from build123d import *

# Parameters (mm, degrees)
CROQUIS1_W                  = 11
CROQUIS1_H                  = 10
SALIENTE_EXTRUIR1_DEPTH     = 4
CROQUIS2_R                  = 0.5
CORTAR_EXTRUIR1_DEPTH       = 12
CROQUIS3_W                  = 8
CROQUIS3_H                  = 1.977477592
CORTAR_EXTRUIR2_DEPTH       = 2
REDONDEO6_R                 = 0.5
REDONDEO8_R                 = 0.5
CORTAR_EXTRUIR3_DEPTH       = 20
CROQUIS5_W                  = 0.5
CROQUIS5_H                  = 1.744690478
CORTAR_EXTRUIR4_DEPTH       = 1
CORTAR_EXTRUIR6_DEPTH       = 12
CORTAR_EXTRUIR6_DEPTH_BACK  = 5
CROQUIS7_W                  = 1
CROQUIS7_H                  = 0.747728434
CROQUIS7_H_2                = 0.24923361
CROQUIS9_W                  = 2
CROQUIS9_H                  = 2
CORTAR_EXTRUIR7_DEPTH       = 1
REDONDEO10_R                = 0.25
CROQUIS11_W                 = 1.5
CROQUIS11_H                 = 1
CROQUIS11_W_2               = 0.5
CROQUIS11_W_3               = 1
REVOLUCI_N5_ANGLE           = 32.23
REVOLUCI_N5_OTHER_WAY_ANGLE = 0.01
CORTAR_EXTRUIR13_DEPTH      = 7
CORTAR_EXTRUIR13_DEPTH_BACK = 10
CROQUIS13_W                 = 2
CROQUIS13_H                 = 2
CORTAR_REVOLUCI_N1_ANGLE    = 5.013380707
CROQUIS15_W                 = 1
CROQUIS15_H                 = 2
REVOLUCI_N6_ANGLE           = 0.716197243
REDONDEO11_R                = 0.5
CROQUIS16_W                 = 2.973519437
CROQUIS16_H                 = 1
CROQUIS16_W_2               = 3
REVOLUCI_N7_ANGLE           = 1.432394488


with BuildPart() as part:
    # Croquis1 → Saliente-Extruir1 (new body)
    with BuildSketch(Plane(origin=(0, 0, 0), x_dir=(1, 0, 0), z_dir=(0, 1, 0))):
        with Locations((44.686928434, -17.152823879)):
            Rectangle(CROQUIS1_W, CROQUIS1_H)
    extrude(amount=SALIENTE_EXTRUIR1_DEPTH)

    # Croquis2 → Cortar-Extruir1 (cut)
    with BuildSketch(Plane.ZY.offset(-39.186928434)):
        with Locations((15.152823879, 2)):
            Circle(CROQUIS2_R)
    extrude(amount=-CORTAR_EXTRUIR1_DEPTH, mode=Mode.SUBTRACT)

    # Croquis3 → Cortar-Extruir2 (cut)
    with BuildSketch(Plane(origin=(0, 4, 0), x_dir=(1, 0, 0), z_dir=(0, 1, 0))):
        with Locations((44.686928434, -20.164085083)):
            Rectangle(CROQUIS3_W, CROQUIS3_H)
    extrude(amount=-CORTAR_EXTRUIR2_DEPTH, mode=Mode.SUBTRACT)

    # Redondeo6
    redondeo6_edges = [part.edges().sort_by_distance(p)[0] for p in [
        (48.686928434, 3, 19.175346287),
        (48.686928434, 3, 21.152823879),
        (40.686928434, 3, 21.152823879),
        (40.686928434, 3, 19.175346287),
    ]]
    fillet(redondeo6_edges, radius=REDONDEO6_R)

    # Redondeo8
    redondeo8_edges = [part.edges().sort_by_distance(p)[0] for p in [
        (44.686928434, 2, 19.175346287),
        (48.686928434, 2, 20.164085083),
        (40.686928434, 2, 20.164085083),
        (44.686928434, 2, 21.152823879),
        (40.833375043, 2, 19.321792897),
        (40.833375043, 2, 21.00637727),
        (48.540481825, 2, 21.00637727),
        (48.540481825, 2, 19.321792897),
    ]]
    fillet(redondeo8_edges, radius=REDONDEO8_R)

    # Croquis4 → Cortar-Extruir3 (cut)
    with BuildSketch(Plane(origin=(50.186928434, 0, 0), x_dir=(0, 0, -1), z_dir=(1, 0, 0))):
        with BuildLine():
            Line((-12.152823879, 4), (-13.897514357, 4))
            ThreePointArc((-13.897514357, 4), (-12.727134054, 3.425689825), (-12.152823879, 2.255309522))
            Line((-12.152823879, 2.255309522), (-12.152823879, 4))
        make_face()
        with BuildLine():
            ThreePointArc((-12.152823879, 1.744690478), (-12.727134054, 0.574310175), (-13.897514357, 0))
            Line((-13.897514357, 0), (-12.152823879, 0))
            Line((-12.152823879, 0), (-12.152823879, 1.744690478))
        make_face()
    extrude(amount=-CORTAR_EXTRUIR3_DEPTH, mode=Mode.SUBTRACT)

    # Croquis5 → Cortar-Extruir4 (cut)
    with BuildSketch(Plane.XZ):
        Polygon((44.686928434, 13.897514357), (44.686928434, 17.970046761), (44.686928434, 20.152823879), (44.186928434, 20.152823879), (44.186928434, 13.897514357), align=None)
        Polygon((44.686928434, 20.152823879), (44.686928434, 17.970046761), (44.686928434, 13.897514357), (45.186928434, 13.897514357), (45.186928434, 20.152823879), align=None)
        with Locations((44.436928434, 13.025169118)):
            Rectangle(CROQUIS5_W, CROQUIS5_H)
        with Locations((44.936928434, 13.025169118)):
            Rectangle(CROQUIS5_W, CROQUIS5_H)
    extrude(amount=-CORTAR_EXTRUIR4_DEPTH, mode=Mode.SUBTRACT)

    # Croquis7 → Cortar-Extruir6 (cut, two sides: drawn at the far end of the back side and taken through both)
    with BuildSketch(Plane.XZ.offset(-1).offset(-CORTAR_EXTRUIR6_DEPTH_BACK)):
        with Locations((44.686928434, 12.775921706)):
            Rectangle(CROQUIS7_W, CROQUIS7_H)
        with Locations((44.686928434, 12.277440684)):
            Rectangle(CROQUIS7_W, CROQUIS7_H_2)
    extrude(amount=CORTAR_EXTRUIR6_DEPTH + CORTAR_EXTRUIR6_DEPTH_BACK, mode=Mode.SUBTRACT)

    # Croquis9 → Cortar-Extruir7 (cut)
    with BuildSketch(Plane.XZ):
        with Locations((44.686928434, 21.152823879)):
            Rectangle(CROQUIS9_W, CROQUIS9_H)
    extrude(amount=-CORTAR_EXTRUIR7_DEPTH, mode=Mode.SUBTRACT)

    # Redondeo10
    redondeo10_edges = [part.edges().sort_by_distance(p)[0] for p in [
        (45.686928434, 0.5, 20.152823879),
        (43.686928434, 0.5, 20.152823879),
    ]]
    fillet(redondeo10_edges, radius=REDONDEO10_R)

    # Croquis11 → Revolución5 (revolve)
    with BuildSketch(Plane.XY.offset(22.152823879)):
        Polygon((39.186928434, 0), (43.686928434, 0), (43.686928434, 1), (42.686928434, 1), (39.686928434, 1), (39.186928434, 1), align=None)
        with Locations((38.436928434, 0.5)):
            Rectangle(CROQUIS11_W, CROQUIS11_H)
        with Locations((38.436928434, 1.5)):
            Rectangle(CROQUIS11_W, CROQUIS11_H)
        with Locations((39.436928434, 1.5)):
            Rectangle(CROQUIS11_W_2, CROQUIS11_H)
        with Locations((43.186928434, 1.5)):
            Rectangle(CROQUIS11_W_3, CROQUIS11_H)
        with Locations((44.186928434, 0.5)):
            Rectangle(CROQUIS11_W_3, CROQUIS11_H)
        with Locations((45.186928434, 0.5)):
            Rectangle(CROQUIS11_W_3, CROQUIS11_H)
        Polygon((45.686928434, 1), (45.686928434, 0), (50.186928434, 0), (50.186928434, 1), (49.686928434, 1), (46.686928434, 1), align=None)
        with Locations((50.936928434, 1.5)):
            Rectangle(CROQUIS11_W, CROQUIS11_H)
        with Locations((49.936928434, 1.5)):
            Rectangle(CROQUIS11_W_2, CROQUIS11_H)
        with Locations((50.936928434, 0.5)):
            Rectangle(CROQUIS11_W, CROQUIS11_H)
        with Locations((46.186928434, 1.5)):
            Rectangle(CROQUIS11_W_3, CROQUIS11_H)
    revolve(axis=Axis((44.686928434, 79, 22.152823879), (-1, 0, 0)), revolution_arc=REVOLUCI_N5_ANGLE)

    # Croquis11 → Revolución5 other way (revolve)
    with BuildSketch(Plane.XY.offset(22.152823879)):
        Polygon((39.186928434, 0), (43.686928434, 0), (43.686928434, 1), (42.686928434, 1), (39.686928434, 1), (39.186928434, 1), align=None)
        with Locations((38.436928434, 0.5)):
            Rectangle(CROQUIS11_W, CROQUIS11_H)
        with Locations((38.436928434, 1.5)):
            Rectangle(CROQUIS11_W, CROQUIS11_H)
        with Locations((39.436928434, 1.5)):
            Rectangle(CROQUIS11_W_2, CROQUIS11_H)
        with Locations((43.186928434, 1.5)):
            Rectangle(CROQUIS11_W_3, CROQUIS11_H)
        with Locations((44.186928434, 0.5)):
            Rectangle(CROQUIS11_W_3, CROQUIS11_H)
        with Locations((45.186928434, 0.5)):
            Rectangle(CROQUIS11_W_3, CROQUIS11_H)
        Polygon((45.686928434, 1), (45.686928434, 0), (50.186928434, 0), (50.186928434, 1), (49.686928434, 1), (46.686928434, 1), align=None)
        with Locations((50.936928434, 1.5)):
            Rectangle(CROQUIS11_W, CROQUIS11_H)
        with Locations((49.936928434, 1.5)):
            Rectangle(CROQUIS11_W_2, CROQUIS11_H)
        with Locations((50.936928434, 0.5)):
            Rectangle(CROQUIS11_W, CROQUIS11_H)
        with Locations((46.186928434, 1.5)):
            Rectangle(CROQUIS11_W_3, CROQUIS11_H)
    revolve(axis=Axis((44.686928434, 79, 22.152823879), (1, 0, 0)), revolution_arc=REVOLUCI_N5_OTHER_WAY_ANGLE)

    # Croquis13 → Cortar-Extruir13 (cut, two sides: drawn at the far end of the back side and taken through both)
    with BuildSketch(Plane(origin=(0, 1, 0), x_dir=(-1, 0, 0), z_dir=(0, -1, 0)).offset(-CORTAR_EXTRUIR13_DEPTH_BACK)):
        with Locations((-44.686928434, -23.139035778)):
            Rectangle(CROQUIS13_W, CROQUIS13_H)
    extrude(amount=CORTAR_EXTRUIR13_DEPTH + CORTAR_EXTRUIR13_DEPTH_BACK, mode=Mode.SUBTRACT)

    # Croquis14 → Cortar-Revolución1 (revolve, cut)
    with BuildSketch(Plane(origin=(0, 32.464000878, 51.49214672), x_dir=(1, 0, 0), z_dir=(0, 0.5333192687106637, 0.8459140367802884))):
        Polygon((39.713408997, -22.987318925), (39.713408997, -23.987318925), (44.700168716, -23.987318925), (44.700168716, -22.987318925), (43.686928434, -22.987318925), (43.686928434, -21.987318925), (42.686928434, -21.987318925), (42.686928434, -22.987318925), align=None)
        Polygon((44.700168716, -22.987318925), (44.700168716, -23.987318925), (49.686928434, -23.987318925), (49.686928434, -22.987318925), (46.686928434, -22.987318925), (46.686928434, -21.987318925), (45.686928434, -21.987318925), (45.686928434, -22.987318925), align=None)
    revolve(axis=Axis((44.700168716, 79, 22.152823879), (1, 0, 0)), revolution_arc=CORTAR_REVOLUCI_N1_ANGLE, mode=Mode.SUBTRACT)

    # Croquis15 → Revolución6 (revolve)
    with BuildSketch(Plane(origin=(0, 32.464000878, 51.49214672), x_dir=(1, 0, 0), z_dir=(0, 0.5333192687106637, 0.8459140367802884))):
        with Locations((37.186928434, -22.987318925)):
            Rectangle(CROQUIS15_W, CROQUIS15_H)
        with Locations((52.186928434, -22.987318925)):
            Rectangle(CROQUIS15_W, CROQUIS15_H)
    revolve(axis=Axis((39.713408997, 79, 22.152823879), (1, 0, 0)), revolution_arc=REVOLUCI_N6_ANGLE)

    # Redondeo11
    # the kernel refuses this fillet: 0.5 mm, written as the material it takes off along each edge
    with BuildSketch(Plane(origin=(52.686928434, 10.585730005, 64.099816155), x_dir=(0, 0.522703953599643, 0.8525142678520415), z_dir=(0, 0.8525142678520415, -0.5227039535996431)), Plane(origin=(52.686928434, 11.115398548, 64.951695193), x_dir=(-1, 0, 0), z_dir=(0, 0.8459140367802884, -0.5333192687106637)), Plane(origin=(36.686928434, 14.42204421, 61.747648364), x_dir=(0, 0.522703953599643, 0.8525142678520415), z_dir=(0, -0.8525142678520415, 0.5227039535996431)), Plane(origin=(36.686928434, 14.922011714, 62.551758484), x_dir=(1, 0, 0), z_dir=(0, -0.8459140367802884, 0.5333192687106637))) as redondeo11_piece_1:
        with BuildLine():
            CenterArc((REDONDEO11_R, -REDONDEO11_R), REDONDEO11_R, 90, 90)
            Line((0, -REDONDEO11_R), (0, 0))
            Line((0, 0), (REDONDEO11_R, 0))
        make_face()
    extrude(amount=4.5, mode=Mode.SUBTRACT)

    # Croquis16 → Revolución7 (revolve)
    with BuildSketch(Plane(origin=(0, 25.534756625, 49.649833864), x_dir=(1, 0, 0), z_dir=(0, 0.4573558931685637, 0.8892837494208389))):
        with Locations((41.200168715, -17.378308347)):
            Rectangle(CROQUIS16_W, CROQUIS16_H)
        with Locations((48.186928434, -17.378308347)):
            Rectangle(CROQUIS16_W_2, CROQUIS16_H)
    revolve(axis=Axis((44.700168716, 79, 22.152823879), (1, 0, 0)), revolution_arc=REVOLUCI_N7_ANGLE)


solid = part.part
Can you work these out from the model? Positions are in its coordinate system, mm. A direction names the side the tool comes from. Coordinates: 2 decimals unless noted, no trailing zeros. Order: outer loops, then holes, each group sorted by start corner. A loop starts at its lowest first (then second) coordinate and runs counter-clockwise, first axis right, second up. Notation, with made-up numbers: M -16,-38 L -9,-38 A17 ccw -9,-25 Z; hole C -32.5,41.25 d1. An arc over 180 degrees is marked long. Answer as CSV lines item,"result".
(1) Suppose I cut it at D-D on z = 17. Please give me the cut outline in (x, y), plus the area to 3 significant figures.
Geometry check:
outline,"M 39.19,0 L 44.19,0 L 44.19,1 L 45.19,1 L 45.19,0 L 50.19,0 L 50.19,4 L 39.19,4 Z"
area,"43.0 mm^2"
(2) Suppose I cut it at B-B on y = 7.5. Please give me the cut outline in (x, z), plus the area to 3 significant figures.
Geometry check:
outline,"M 37.69,50.73 L 39.69,50.73 L 39.69,53.33 L 42.69,53.33 L 42.69,50.73 L 43.69,50.73 L 43.69,53.33 L 45.69,53.33 L 45.69,50.73 L 46.69,50.73 L 46.69,53.33 L 49.69,53.33 L 49.69,50.73 L 51.69,50.73 L 51.69,55.75 L 37.69,55.75 Z"
area,"49.5 mm^2"
(3) On a 3-axis mill with a long thin cutter (end or side, diameter ignored), from which of +Z, -Z, +X, -X, +Y, -Y can I reach the whole of each face in a straight line? I mean faces 1 (the flat face through (48, 2, 22.153)), 2 (the flat face through (44.187, 0.8, 15.6)), 3 (the flat face through (45, 2, 13.15)). Say none if no direction works.
Geometry check:
face 1,"+Y"
face 2,"-Z, -Y"
face 3,"-Z, +Y, -Y"
(4) I'm going to push flat-ended pins straight in: pin 1 (3 mm diameter, centred on y = 4, z = 36, fed in from -X); pin 2 (4 mm diameter, centred on y = 2.5, z = 25, fed in from +X); pin 3 (2 mm diameter, centred on x = 43, z = 32, fed in from -Y). Where does each tip first touch, or does it pass through?
Geometry check:
pin 1,"x = 37.69"
pin 2,"x = 51.69"
pin 3,"y = 0.5"
(5) If we mould it in two halves opening along X, with no side actions, what happens to faces 4 (the flat face through (45.687, 3.7, 39)), 5 (the flat face through (45, 4, 17))? For each: released by +X, released by -X, zero draft, split by the parting line, or undercut.
Geometry check:
face 4,"undercut"
face 5,"zero draft"
(6) Please list where these lines run through material, in increasing order: L1, parallel to X at y = 4, z = 43; L2, parallel to X at y = 3, z = 22; L3, parallel to Y at x = 42, z = 15.
Geometry check:
L1,"37.69 to 39.69, 42.69 to 43.69, 45.69 to 46.69, 49.69 to 51.69"
L2,"39.19 to 50.19"
L3,"0 to 1.52, 2.48 to 4"
(7) Suppose I cut it at A-A on x = 47.5. Please give me the cut outline in (y, z).
Geometry check:
outline,"M 0,13.9 A2.02 ccw 1.74,12.15 L 2.26,12.15 A2.02 ccw 4,13.9 L 4,19.18 L 2.5,19.18 A0.5 cw 2,19.68 L 2,20.65 A0.5 cw 2.5,21.15 L 4,21.15 L 4,22.15 L 1,22.15 A78 cw 8.77,56.08 L 9.67,55.65 A77 cw 10.53,57.37 L 8.75,58.28 A79 ccw 0,22.15 Z; hole C 2,15.15 d1"
(8) Suppose I cut it at C-C on z = 39. Please give me the cut outline in (x, y).
Geometry check:
outline,"M 37.69,1.82 L 51.69,1.82 L 51.69,3.87 L 49.69,3.87 L 49.69,2.84 L 46.69,2.84 L 46.69,3.87 L 45.69,3.87 L 45.69,2.84 L 43.69,2.84 L 43.69,3.87 L 42.69,3.87 L 42.69,2.84 L 39.69,2.84 L 39.69,3.87 L 37.69,3.87 Z"
